The model under review builds one solid part; all positions refer to its coordinate system, in mm. A direction names the side the tool comes from. Round coordinates to 2 decimals unless told otherwise and drop trailing zeros. Loops run counter-clockwise (first coordinate to the right, second up) from the corner with the lowest first, then second, coordinate; pieces in that order, holes last. Notation, with made-up numbers: M 48,43 L 72,43 A20 cw 72,52 Z; hole C -29.75,-34.5 d5. An arc over 180 degrees is marked long. Return JSON: item names as keys, results as strings. Group by question number.
Q1. To check wall thickness, follow line 1 along Z through (x, y) = (0, 3.25); line 2 along Z through (x, y) = (-1, -0.5) (3 decimals); line 3 along X through (y, z) = (1.5, -6). State the ranges of each line that lie inside material, in increasing order.
Q2. Clearance check with flat-ended pins moving along their axes: pin 1 Ø1.5 at (x, z) = (0, -5) entering from -Y; pin 2 Ø1.5 at (x, z) = (-3, -6.5) entering from -Y; pin 3 Ø3 at (x, y) = (2, 3) entering from -Z; pin 4 Ø1.5 at (x, z) = (-1, -2.5) entering from +Y. State where each tip first meets the part, or that it passes through.
Q3. Consider section A-A (z = -5.5). State the section outline as (x, y) points, and give its area (3 significant figures).
Q4. For faces 1 (the face through (0, 0, -9.525)), 2 (the face through (-0.43, 1.937, -4.954)), list the 3-axis set-ups (+Z, -Z, +X, -X, +Y, -Y) from which the entire face can be reached by the end or side of a thin tool; tool diameter is ignored.
from build123d import *

# Parameters (mm, degrees)
CUT_EXTRUDE1_DEPTH      = 22.542442188
CUT_EXTRUDE1_DEPTH_BACK = 22.542442188
CUT_EXTRUDE2_DEPTH      = 22.542442188
CUT_EXTRUDE2_DEPTH_BACK = 22.542442188
FILLET2_R               = 0.254
LPATTERN1_COUNT         = 18
LPATTERN1_PITCH         = 0.762
CUT_EXTRUDE3_DEPTH      = 22.542442285
CUT_EXTRUDE3_DEPTH_BACK = 22.542442285
SKETCH7_W               = 2.637927388
SKETCH7_H               = 20.320175892


with BuildPart() as part:
    # Sketch2 → Revolve1 (revolve)
    with BuildSketch(Plane(origin=(0, 0, 0), x_dir=(0, 0, -1), z_dir=(1, 0, 0)), mode=Mode.PRIVATE) as revolve1_sk:
        with BuildLine():
            Line((-20.7264, 0), (-20.7264, 0.9921875))
            Line((-20.7264, 0.9921875), (-1.6764, 0.9921875))
            ThreePointArc((-1.6764, 0.9921875), (-1.282773396, 2.741180458), (-0.1778, 4.1529))
            Line((-0.1778, 4.1529), (0, 4.1529))
            Line((0, 4.1529), (0, 1.984375))
            Line((0, 1.984375), (9.525, 1.984375))
            Line((9.525, 1.984375), (9.525, 1.870886692))
            Line((9.525, 1.870886692), (9.525, 0))
            Line((9.525, 0), (-20.7264, 0))
        make_face()
    revolve(revolve1_sk.sketch.rotate(Axis((0, 0, 20.7264), (0, 0, -1)), 90), axis=Axis((0, 0, 20.7264), (0, 0, -1)))

    # Sketch3 → Cut-Extrude1 (cut, two sides: drawn at the far end of the back side and taken through both)
    with BuildSketch(Plane(origin=(0, 0, 0), x_dir=(1, 0, 0), z_dir=(0, 1, 0)).offset(-CUT_EXTRUDE1_DEPTH_BACK)):
        Polygon((0, -20.7264), (1.1953875, -19.16854068), (1.1953875, -21.2344), (-1.1953875, -21.2344), (-1.1953875, -19.16854068), align=None)
    extrude(amount=CUT_EXTRUDE1_DEPTH + CUT_EXTRUDE1_DEPTH_BACK, mode=Mode.SUBTRACT)

    # Sketch5 → Cut-Extrude2 (cut, two sides: drawn at the far end of the back side and taken through both)
    with BuildSketch(Plane(origin=(0, 0, 0), x_dir=(0, 0, -1), z_dir=(1, 0, 0)).offset(-CUT_EXTRUDE2_DEPTH_BACK)):
        Polygon((-20.7264, 0), (-19.433356075, 1.3096875), (-21.0439, 1.3096875), (-21.0439, -1.3096875), (-19.433356075, -1.3096875), align=None)
    extrude(amount=CUT_EXTRUDE2_DEPTH + CUT_EXTRUDE2_DEPTH_BACK, mode=Mode.SUBTRACT)

    # Fillet2
    fillet2_edges = [part.edges().sort_by_distance(p)[0] for p in [
        (-1.984375, 0, 0),
    ]]
    fillet(fillet2_edges, radius=FILLET2_R)

    # Sketch6 → Cut-Revolve1 (revolve, cut)
    with BuildSketch(Plane(origin=(0, 0, 0), x_dir=(0, 0, -1), z_dir=(1, 0, 0)), mode=Mode.PRIVATE) as cut_revolve1_sk:
        with BuildLine():
            Line((-6.5913, 0.9921875), (-6.4389, 0.9921875))
            ThreePointArc((-6.4389, 0.9921875), (-6.5151, 0.9159875), (-6.5913, 0.9921875))
        make_face()
    cut_revolve1 = revolve(cut_revolve1_sk.sketch.rotate(Axis((0, 0, 20.7264), (0, 0, -1)), 90), axis=Axis((0, 0, 20.7264), (0, 0, -1)), mode=Mode.SUBTRACT)

    # LPattern1: Cut-Revolve1 ×18
    with Locations(*[(0, 0, i * LPATTERN1_PITCH) for i in range(1, LPATTERN1_COUNT)]):
        add(cut_revolve1, mode=Mode.SUBTRACT)

    # Sketch7 → Cut-Extrude3 (cut, two sides: drawn at the far end of the back side and taken through both)
    with BuildSketch(Plane(origin=(0, 0, 0), x_dir=(1, 0, 0), z_dir=(0, 1, 0)).offset(-CUT_EXTRUDE3_DEPTH_BACK)):
        with Locations((0.326776194, -11.836487946)):
            Rectangle(SKETCH7_W, SKETCH7_H)
    extrude(amount=CUT_EXTRUDE3_DEPTH + CUT_EXTRUDE3_DEPTH_BACK, mode=Mode.SUBTRACT)


solid = part.part
Values:
{
 "1": {"line 1": "z = 0 to 1", "line 2": "z = -9.525 to 1.674", "line 3": "x = -1.3 to 1.3"},
 "2": {"pin 1": "stops at y = -1.98", "pin 2": "passes through", "pin 3": "stops at z = -0.04", "pin 4": "stops at y = 1.97"},
 "3": {"outline": "C 0,0 d3.97", "area": "12.4 mm2"},
 "4": {"face 1": "-Z, +X, -X, +Y, -Y", "face 2": "-Z"}
}
